```python
from build123d import *

# Parameters (mm, degrees)
SKETCH_1_R          = 1.5
SKETCH_1_W          = 39
SKETCH_1_H          = 12.5
EXTRUDE_1_DEPTH     = 2
SKETCH_2_R          = 1
SKETCH_2_W          = 29
SKETCH_2_H          = 20.7
CUT_EXTRUDE_1_DEPTH = 65.231534311
FILLET_1_R          = 1


with BuildPart() as part:
    # 草图1 → 凸台-拉伸1 (new body)
    with BuildSketch(Plane(origin=(0, 0, 0), x_dir=(1, 0, 0), z_dir=(0, 1, 0))):
        Polygon((-22.5, 3), (-22.5, 33.2), (-26, 33.2), (-26, 58.7), (26, 58.7), (26, 33.2), (22.5, 33.2), (22.5, 3), (12.5, 3), (12.5, 0), (-12.5, 0), (-12.5, 3), align=None)
        with Locations(Location((-22.5, 55.2, 0), (0, 0, 270))):
            Circle(SKETCH_1_R, mode=Mode.SUBTRACT)
        with Locations(Location((-22.5, 36.7, 0), (0, 0, 270))):
            Circle(SKETCH_1_R, mode=Mode.SUBTRACT)
        with Locations(Location((22.5, 36.7, 0), (0, 0, 90))):
            Circle(SKETCH_1_R, mode=Mode.SUBTRACT)
        with Locations(Location((22.5, 55.2, 0), (0, 0, 90))):
            Circle(SKETCH_1_R, mode=Mode.SUBTRACT)
        with Locations(Location((-17.5, 8, 0), (0, 0, 270))):
            Circle(SKETCH_1_R, mode=Mode.SUBTRACT)
        with Locations(Location((17.5, 8, 0), (0, 0, 90))):
            Circle(SKETCH_1_R, mode=Mode.SUBTRACT)
        with Locations((0, 45.95)):
            Rectangle(SKETCH_1_W, SKETCH_1_H, mode=Mode.SUBTRACT)
    extrude(amount=EXTRUDE_1_DEPTH)

    # 草图2 → 切除-拉伸1 (cut, through all)
    with BuildSketch(Plane(origin=(0, 2, 0), x_dir=(1, 0, 0), z_dir=(0, 1, 0))):
        with Locations((-13.5, 3)):
            Circle(SKETCH_2_R)
        with Locations((13.5, 3)):
            Circle(SKETCH_2_R)
        with Locations((0, 23.35)):
            Rectangle(SKETCH_2_W, SKETCH_2_H)
    extrude(amount=-CUT_EXTRUDE_1_DEPTH, mode=Mode.SUBTRACT)

    # 圆角1
    fillet_1_edges = [part.edges().sort_by_distance(p)[0] for p in [
        (26, 1, -33.2),
        (22.5, 1, -33.2),
        (22.5, 1, -3),
        (12.5, 1, 0),
        (-12.5, 1, 0),
        (-22.5, 1, -3),
        (-22.5, 1, -33.2),
        (-26, 1, -33.2),
        (-26, 1, -58.7),
        (26, 1, -58.7),
        (-19.5, 1, -52.2),
        (-19.5, 1, -39.7),
        (19.5, 1, -39.7),
        (19.5, 1, -52.2),
        (-14.5, 1, -13),
        (-14.5, 1, -33.7),
        (14.5, 1, -33.7),
        (14.5, 1, -13),
    ]]
    fillet(fillet_1_edges, radius=FILLET_1_R)


solid = part.part
```
Input: part model. Units: mm. Frame: model coordinates. A direction names the side the tool comes from. Coordinates: 2 decimals unless noted, no trailing zeros. Loops run counter-clockwise (first coordinate to the right, second up) from the corner with the lowest first, then second, coordinate; pieces in that order, holes last.
Q1. Section B-B, the plane x = -17.5. Return the cut outline in (y, z), and give its area (3 significant figures).
Results are:
outline: (0, -58.7) - (2, -58.7) - (2, -52.2) - (0, -52.2) - close; (0, -39.7) - (2, -39.7) - (2, -9.5) - (0, -9.5) - close; (0, -6.5) - (2, -6.5) - (2, -3) - (0, -3) - close
area: 80.4 mm2
Q2. Line query: line 1 along Z through (x, y) = (0.5, 0.25); line 2 along X through (y, z) = (1.5, -8); line 3 along X through (y, z) = (0.65, -36.7). Output: solid intervals per line, ascending.
Results are:
line 1: z = -58.7 to -52.2, -39.7 to -33.7, -13 to 0
line 2: x = -22.5 to -19, -16 to 16, 19 to 22.5
line 3: x = -26 to -24, -21 to 21, 24 to 26
Q3. Section D-D, the plane z = -44. Return the cut outline in (x, y).
Results are:
outline: (-26, 0) - (-19.5, 0) - (-19.5, 2) - (-26, 2) - close; (19.5, 0) - (26, 0) - (26, 2) - (19.5, 2) - close
Q4. Section A-A, the plane z = -17. Return the cut outline in (x, y).
Results are:
outline: (-22.5, 0) - (-14.5, 0) - (-14.5, 2) - (-22.5, 2) - close; (14.5, 0) - (22.5, 0) - (22.5, 2) - (14.5, 2) - close
Q5. Contact query for flat-ended pins moving along their axis: pin 1 (0.6 mm diameter, centred on y = 1, z = -14, fed in from +X); pin 2 (0.6 mm diameter, centred on y = 1.5, z = -2, fed in from +X). Output: stop coordinate, or through.
Results are:
pin 1: stops at x = 22.5
pin 2: stops at x = 12.5
Q6. Set-up query: faces 4 (the flat face through (14.5, 1, -23)), 5 (the flat face through (24, 1, -33.2)), 6 (the flat face through (-12.5, 1, -2)). Return all of +Z, -Z, +X, -X, +Y, -Y with unobstructed straight access to the full face (end or side cutting, diameter ignored); none if empty.
Results are:
face 4: +Y, -Y
face 5: +Z, +X, +Y, -Y
face 6: +Z, -X, +Y, -Y
Q7. Mould query, pull axis X, two halves, no side actions, for faces 1 (the flat face through (0, 1, -33.7)), 2 (the flat face through (26, 1, -46)), 3 (the flat face through (-22.5, 1, -18)). Classes: +X half, -X half, draft (parallel to the pull), parting line (faces both ways), or undercut.
Results are:
face 1: undercut
face 2: +X half
face 3: -X half
Q8. Section C-C, the plane z = -55.2. Return the cut outline in (x, y).
Results are:
outline: (-26, 0) - (-24, 0) - (-24, 2) - (-26, 2) - close; (-21, 0) - (21, 0) - (21, 2) - (-21, 2) - close; (24, 0) - (26, 0) - (26, 2) - (24, 2) - close
